from build123d import *

# Parameters (mm, degrees)
BOSS_EXTRUDE1_DEPTH = 25.4
SKETCH2_R           = 1.99898
CUT_EXTRUDE1_DEPTH  = 25.4


with BuildPart() as part:
    # Sketch1 → Boss-Extrude1 (new body)
    with BuildSketch(Plane(origin=(0, 0, 0), x_dir=(1, 0, 0), z_dir=(0, 1, 0))):
        with BuildLine():
            Line((0, 0), (203.2, 0))
            Line((203.2, 0), (203.2, 25.4))
            ThreePointArc((203.2, 25.4), (177.8, 50.8), (152.4, 25.4))
            Line((152.4, 25.4), (0, 25.4))
            Line((0, 25.4), (0, 0))
        make_face()
    extrude(amount=BOSS_EXTRUDE1_DEPTH)

    # Sketch2 → Cut-Extrude1 (cut)
    with BuildSketch(Plane(origin=(0, 25.4, 0), x_dir=(1, 0, 0), z_dir=(0, 1, 0))):
        with Locations(Location((10.16, 12.7, 0), (0, 0, 270))):
            Circle(SKETCH2_R)
        with Locations(Location((18.4658, 12.7, 0), (0, 0, 270))):
            Circle(SKETCH2_R)
    extrude(amount=-CUT_EXTRUDE1_DEPTH, mode=Mode.SUBTRACT)


solid = part.part
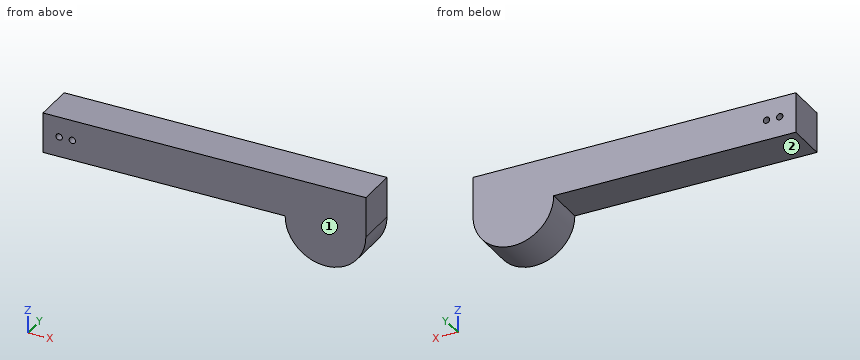
Here's how the part is built. I have some questions about the finished solid (model axes, mm). Face numbers are marked on the shaded views. A direction names the side the tool comes from. Coordinates: 2 decimals unless noted, no trailing zeros. Order: outer loops, then holes, each group sorted by start corner. A loop starts at its lowest first (then second) coordinate and runs counter-clockwise, first axis right, second up. Notation, with made-up numbers: M -25,0 L 28,0 A17 ccw 28,12 Z; hole C 68.5,-21.5 d7. An arc over 180 degrees is marked long. Answer as CSV lines item,"result". Start each with the question number.
1. I want a section at B-B, the plane z = -12.7. Write out the boundary of the cut face in (x, y), and give its area (3 significant figures).
2. I want a section at C-C, the plane y = 14.75. Write out the boundary of the cut face in (x, z), and give its area (3 significant figures).
3. I need wall thicknesses on line 1 (X direction, y = 16, z = -11); line 2 (Z direction, x = 117, y = 4); line 3 (X direction, y = 18.75, z = -35). Which ranges of each line are inside material? Lowest first, please. Write a range as [from, to].
4. On a 3-axis mill with a long thin cutter (end or side, diameter ignored), from which of +Z, -Z, +X, -X, +Y, -Y can I reach the whole of each face in a straight line? I mean the marked faces 1 and 2. Say none if no direction works.
5. I want a section at D-D, the plane x = 127. Write out the boundary of the cut face in (y, z), and give its area (3 significant figures).
6. For pin 1 (2.5 mm diameter, centred on x = 10.16, z = -12.7, fed in from -Y); pin 2 (3 mm diameter, centred on x = 64, y = 20.5, fed in from -Z), each with a flat end and sliding along its axis, tell me the tip position at first contact or that it passes through.
7. I want a section at A-A, the plane x = 10.16. Write out the boundary of the cut face in (y, z), and give its area (3 significant figures).
Recorded:
1,outline,"M 0,0 L 8.16,0 L 8.16,25.4 L 0,25.4 Z; M 12.16,0 L 16.47,0 L 16.47,25.4 L 12.16,25.4 Z; M 20.46,0 L 203.2,0 L 203.2,25.4 L 20.46,25.4 Z"
1,area,"4,960 mm2"
2,outline,"M 0,-25.4 L 152.4,-25.4 A25.4 ccw 203.2,-25.4 L 203.2,0 L 0,0 Z; hole C 10.16,-12.7 d4; hole C 18.47,-12.7 d4"
2,area,"6,150 mm2"
3,line 1,"x = [0, 9.11], [11.21, 17.41], [19.52, 203.2]"
3,line 2,"z = [-25.4, 0]"
3,line 3,"x = [154.28, 201.32]"
4,face 1,"+Z, -Z, +X, -X, -Y"
4,face 2,"-Z, -X, +Y, -Y"
5,outline,"M 0,-25.4 L 25.4,-25.4 L 25.4,0 L 0,0 Z"
5,area,"645 mm2"
6,pin 1,"passes through"
6,pin 2,"stops at z = -25.4"
7,outline,"M 0,-25.4 L 25.4,-25.4 L 25.4,-14.7 L 0,-14.7 Z; M 0,-10.7 L 25.4,-10.7 L 25.4,0 L 0,0 Z"
7,area,"544 mm2"
